Part model, mm, in its own coordinate system. Round coordinates to 2 decimals unless told otherwise and drop trailing zeros. Write each loop counter-clockwise with the first axis right and the second up, starting at its lowest first coordinate (ties: lowest second). Pieces come first, ordered by that corner, then holes. Notation, with made-up numbers: (14, 57.25) -> (35, 57.25) arc R15 ccw to (35, 84.25) -> close; hole circle Ø10 at (10.25, 14.5). An arc over 180 degrees is marked (long way). Return JSON: item names as keys, results as strings. Group by question number.
(1) Drill centre lines: L1, parallel to Y at x = -70, z = 0.3; L2, parallel to Y at x = 58.5, z = 0.95; L3, parallel to Y at x = 80.5, z = 0.7. Where is each one in solid material? Low to high. Write a range as from..to.
(2) Mould opens along Y. For faces 1 (the cylindrical face through (60.79, -44.55, 0.49)), 2 (the flat face through (63, 29, 1)), 3 (the flat face through (-88, 81, 0.5)) say: +Y half, -Y half, draft (parallel to the pull), parting line (faces both ways), or undercut.
(3) Saw through at A-A (x = 0). List the corners of the cut face in (y, z).
(4) Saw through at C-C (z = 0.15). State how many separate pieces and enclosed holes the cut face has, plus the area to 3 significant figures.
(5) Saw through at D-D (y = -53). List the corners of the cut face in (x, z).
(6) Saw through at B-B (y = 0). List the corners of the cut face in (x, z), plus the area to 3 significant figures.
(7) Drop a flat-ended pin along its axis: pin 1 Ø8 at (x, y) = (2, 78) entering from -Z. Give the stop position or say it passes through.
from build123d import *

# Parameters (mm, degrees)
SKETCH1_R      = 6.5
SKETCH1_R_2    = 68.7
SKETCH1_R_3    = 12.5
EXTRUDE1_DEPTH = 1
FILLET1_R      = 10
FILLET2_R      = 3


with BuildPart() as part:
    # Sketch1 → Extrude1 (new body)
    with BuildSketch(Plane.XY):
        Polygon((84, 85), (92, 77), (92, -77), (84, -86), (-84, -86), (-92, -77), (-92, 77), (-84, 85), (-19.8, 85), (-12.75, 100), (12.75, 100), (19.8, 85), align=None)
        with Locations(Location((-78, -24.5, 0), (0, 0, 180))):
            Circle(SKETCH1_R, mode=Mode.SUBTRACT)
        Circle(SKETCH1_R_2, mode=Mode.SUBTRACT)
        with Locations((-70, 62)):
            Circle(SKETCH1_R_3, mode=Mode.SUBTRACT)
        with Locations((70, 62)):
            Circle(SKETCH1_R_3, mode=Mode.SUBTRACT)
        with Locations((-70, -53)):
            Circle(SKETCH1_R_3, mode=Mode.SUBTRACT)
        with Locations((70, -53)):
            Circle(SKETCH1_R_3, mode=Mode.SUBTRACT)
        with Locations((78, -24.5)):
            Circle(SKETCH1_R, mode=Mode.SUBTRACT)
    extrude(amount=EXTRUDE1_DEPTH)

    # Fillet1
    fillet1_edges = [part.edges().sort_by_distance(p)[0] for p in [
        (-19.8, 85, 0.5),
        (19.8, 85, 0.5),
    ]]
    fillet(fillet1_edges, radius=FILLET1_R)

    # Fillet2
    fillet2_edges = [part.edges().sort_by_distance(p)[0] for p in [
        (92, -77, 0.5),
        (84, -86, 0.5),
        (-84, -86, 0.5),
        (-92, -77, 0.5),
        (-92, 77, 0.5),
        (-84, 85, 0.5),
        (-12.75, 100, 0.5),
        (12.75, 100, 0.5),
        (84, 85, 0.5),
        (92, 77, 0.5),
    ]]
    fillet(fillet2_edges, radius=FILLET2_R)


solid = part.part
Computed values:
{
 "1": {"L1": "-86..-65.5, -40.5..49.5, 74.5..85", "L2": "-86..-57.9, -48.1..-36.02, 36.02..57.1, 66.9..85", "L3": "-86..-59.78, -46.22..-30.5, -18.5..55.22, 68.78..85"},
 "2": {"face 1": "undercut", "face 2": "draft", "face 3": "+Y half"},
 "3": {"outline": "(-86, 0) -> (-68.7, 0) -> (-68.7, 1) -> (-86, 1) -> close; (68.7, 0) -> (100, 0) -> (100, 1) -> (68.7, 1) -> close"},
 "4": {"separate pieces": "1", "enclosed holes": "7", "area": "14,800 mm2"},
 "5": {"outline": "(-92, 0) -> (-82.5, 0) -> (-82.5, 1) -> (-92, 1) -> close; (-57.5, 0) -> (-43.71, 0) -> (-43.71, 1) -> (-57.5, 1) -> close; (43.71, 0) -> (57.5, 0) -> (57.5, 1) -> (43.71, 1) -> close; (82.5, 0) -> (92, 0) -> (92, 1) -> (82.5, 1) -> close"},
 "6": {"outline": "(-92, 0) -> (-68.7, 0) -> (-68.7, 1) -> (-92, 1) -> close; (68.7, 0) -> (92, 0) -> (92, 1) -> (68.7, 1) -> close", "area": "46.6 mm2"},
 "7": {"pin 1": "z = 0"}
}
